Part print with two shaded views. Sizes in mm from the minimum x, y, z corner. Give positions to 0.01 mm unless a question says otherwise; leave off trailing zeros. Write each loop counter-clockwise with the first axis right and the second up, starting at its lowest first coordinate (ties: lowest second). Pieces come first, ordered by that corner, then holes.
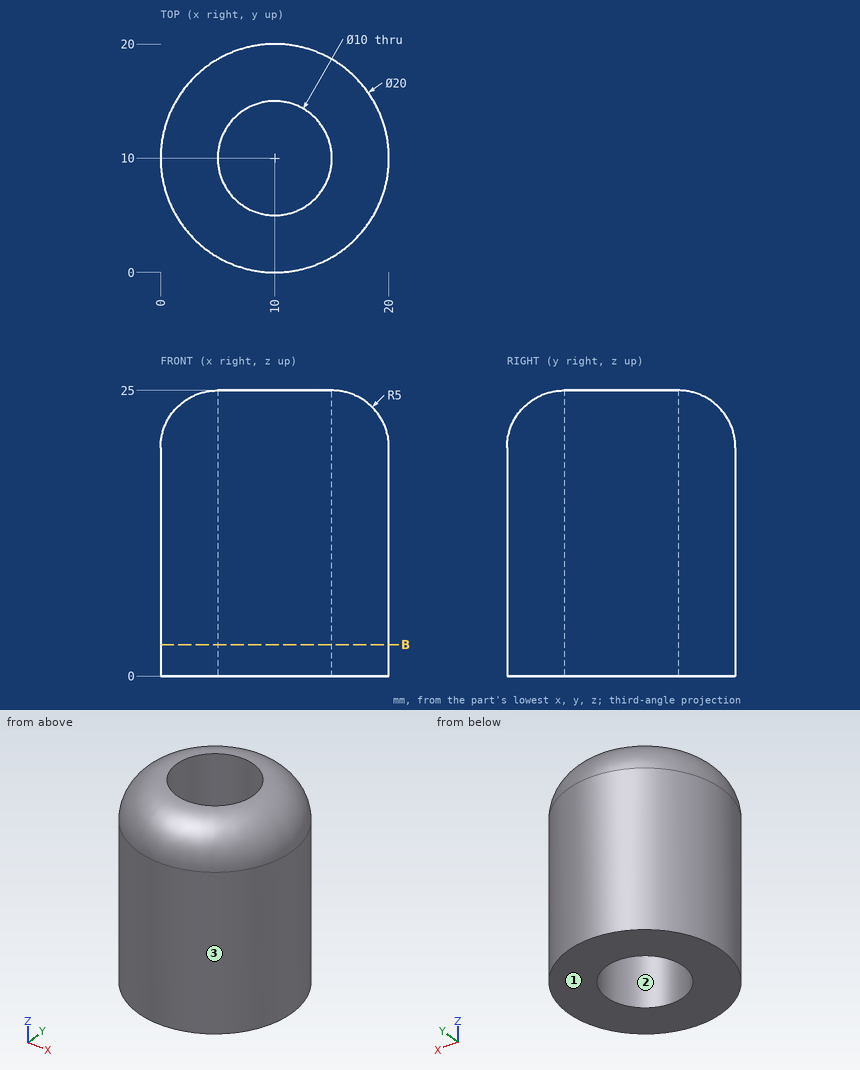
1) Wall check: L1, parallel to Y at x = 10, z = 17.75; L2, parallel to X at y = 10.75, z = 4.5; L3, parallel to X at y = 11.5, z = 14.75. Give the ranges that are in metal, low to high.
Answers follow:
L1: y = 0 to 5, 15 to 20
L2: x = 0.03 to 5.06, 14.94 to 19.97
L3: x = 0.11 to 5.23, 14.77 to 19.89
2) Saw through at B-B, the plane z = 2.75. Write the cut outline in (x, y), then the cut area to 3 significant figures.
Answers follow:
outline: circle Ø20 at (10, 10); hole circle Ø10 at (10, 10)
area: 236 mm2
3) Two-plate mould, pull along X, no slides. Class the marked faces 1, 2 and 3: +X half, -X half, draft (parallel to the pull), parting line (faces both ways), or undercut.
Answers follow:
face 1: draft
face 2: undercut
face 3: parting line
